Source: CAD feature listing. Evaluate the final solid. Frame: model axes, mm. Face numbers are marked on the shaded views. Coordinates: 2 decimals unless noted, no trailing zeros. Order: outer loops, then holes, each group sorted by start corner. A loop starts at its lowest first (then second) coordinate and runs counter-clockwise, first axis right, second up.
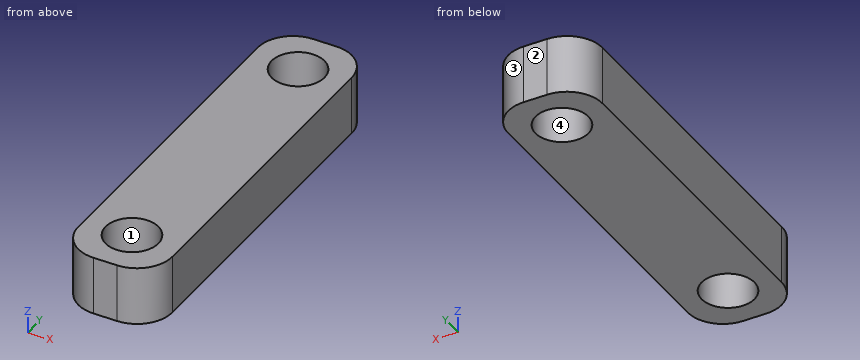
```python
from build123d import *

# Parameters (mm, degrees)
SKETCH1_W           = 8
SKETCH1_H           = 33
SKETCH1_R           = 2.25
BOSS_EXTRUDE1_DEPTH = 5
FILLET1_R           = 3


with BuildPart() as part:
    # Sketch1 → Boss-Extrude1 (new body)
    with BuildSketch(Plane.XY):
        with Locations((4, -16.5)):
            Rectangle(SKETCH1_W, SKETCH1_H)
        with Locations((4, -29)):
            Circle(SKETCH1_R, mode=Mode.SUBTRACT)
        with Locations((4, -4)):
            Circle(SKETCH1_R, mode=Mode.SUBTRACT)
    extrude(amount=BOSS_EXTRUDE1_DEPTH)

    # Fillet1
    fillet1_edges = [part.edges().sort_by_distance(p)[0] for p in [
        (0, 0, 2.5),
        (8, 0, 2.5),
        (8, -33, 2.5),
        (0, -33, 2.5),
    ]]
    fillet(fillet1_edges, radius=FILLET1_R)


solid = part.part
```
1. Section query D-D, the plane x = 2.5. Output: boundary loops of the cut face in (y, z), plus the area to 3 significant figures.
2. Section query C-C, the plane x = 4. Output: boundary loops of the cut face in (y, z), plus the area to 3 significant figures.
3. Section query B-B, the plane y = -4. Output: boundary loops of the cut face in (x, z), plus the area to 3 significant figures.
4. Contact query for flat-ended pins moving along their axis: P1, Ø3, axis at x = 1, y = -8.5, coming from the -Z side; P2, Ø4, axis at x = 4, y = -4, coming from the -Z side. Output: stop coordinate, or through.
5. Draft query along X for the marked faces 1, 2, 3 and 4. Return one class per face: +X half, -X half, draft (parallel to the pull), parting line (faces both ways), or undercut.
6. Section query A-A, the plane z = 4.25. Output: boundary loops of the cut face in (x, y).
7. Material intervals for line 1 along Y through (x, z) = (4, 2.8); line 2 along Y through (x, z) = (5.75, 1.7); line 3 along X through (y, z) = (-30.5, 4), sorted ascending.
Answer key:
1. outline: (-32.96, 0) - (-30.68, 0) - (-30.68, 5) - (-32.96, 5) - close; (-27.32, 0) - (-5.68, 0) - (-5.68, 5) - (-27.32, 5) - close; (-2.32, 0) - (-0.04, 0) - (-0.04, 5) - (-2.32, 5) - close
1. area: 131 mm2
2. outline: (-33, 0) - (-31.25, 0) - (-31.25, 5) - (-33, 5) - close; (-26.75, 0) - (-6.25, 0) - (-6.25, 5) - (-26.75, 5) - close; (-1.75, 0) - (0, 0) - (0, 5) - (-1.75, 5) - close
2. area: 120 mm2
3. outline: (0, 0) - (1.75, 0) - (1.75, 5) - (0, 5) - close; (6.25, 0) - (8, 0) - (8, 5) - (6.25, 5) - close
3. area: 17.5 mm2
4. P1: stops at z = 0
4. P2: passes through
5. face 1: undercut
5. face 2: draft
5. face 3: +X half
5. face 4: undercut
6. outline: (0, -30) arc R3 ccw to (3, -33) - (5, -33) arc R3 ccw to (8, -30) - (8, -3) arc R3 ccw to (5, 0) - (3, 0) arc R3 ccw to (0, -3) - close; hole circle Ø4.5 at (4, -29); hole circle Ø4.5 at (4, -4)
7. line 1: y = -33 to -31.25, -26.75 to -6.25, -1.75 to 0
7. line 2: y = -32.9 to -30.41, -27.59 to -5.41, -2.59 to -0.1
7. line 3: x = 0.04 to 2.32, 5.68 to 7.96
